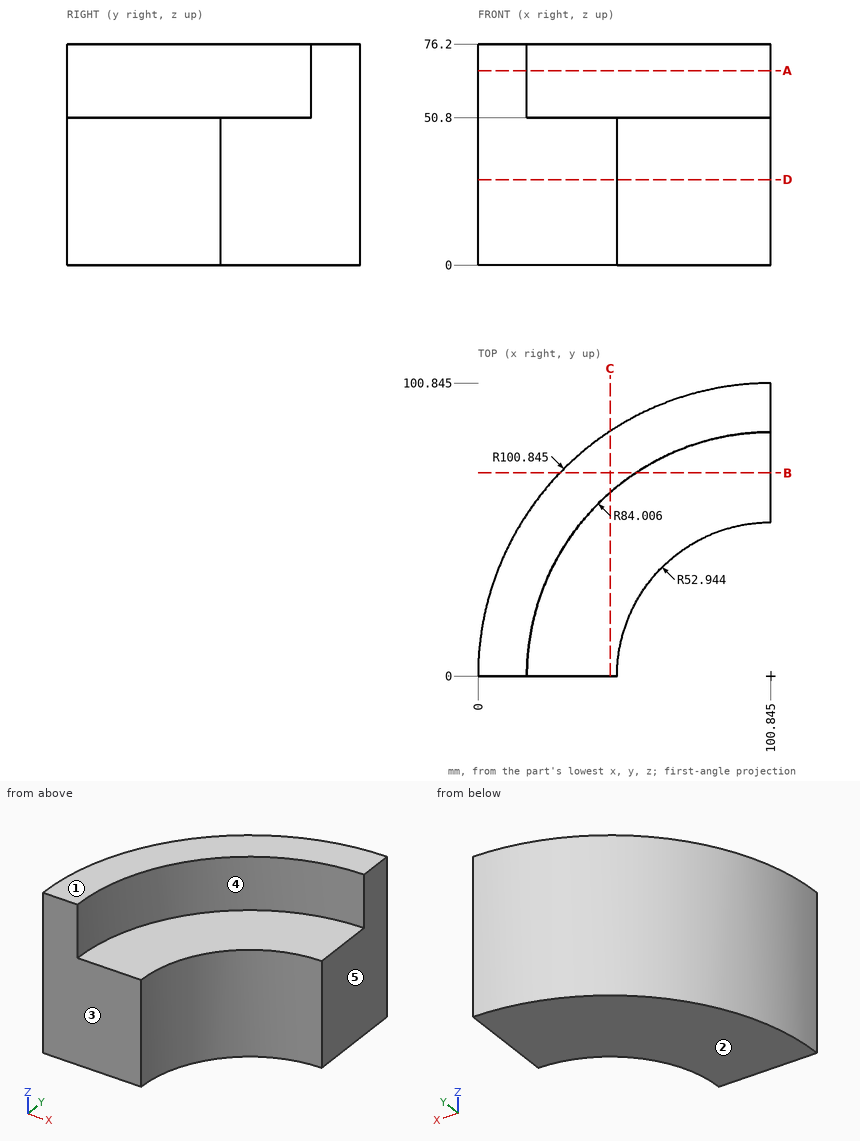
Can you work these out from the drawing? Everything is in mm from the part's minimum corner. A direction names the side the tool comes from. Round coordinates to 2 decimals unless told otherwise and drop trailing zeros. Write each loop counter-clockwise with the first axis right and the second up, starting at its lowest first coordinate (ties: lowest second). Pieces come first, ordered by that corner, then holes.
1. If we mould it in two halves opening along Z, with no side actions, what happens to the marked faces 1, 2 and 3? For each: released by +Z, released by -Z, zero draft, split by the parting line, or undercut.
2. For the marked faces 4 and 5, which set-ups out of +Z, -Z, +X, -X, +Y, -Y let a thin tool reach every point of the face, with its end or its side?
3. Suppose I cut it at C-C (x = 45.5). List the corners of the cut face in (y, z) for me.
4. Will these pins go through, and if not, where does the flat tip stop? pin 1 Ø1 at (x, y) = (50.5, 34) entering from +Z; pin 2 Ø4 at (y, z) = (67, 67) entering from +X; pin 3 Ø4 at (y, z) = (80.5, 39.5) entering from -X; pin 4 Ø25 at (x, y) = (38, 35) entering from +Z.
5. I need wall thicknesses on L1, parallel to Z at x = 59, y = 58; L2, parallel to Y at x = 68, z = 69 (1 decimal); L3, parallel to Y at x = 25.5, z = 27. Which ranges of each line are inside material? Lowest first, please.
6. Suppose I cut it at A-A (z = 67). List the corners of the cut face in (x, y) for me (1 decimal).
7. Suppose I cut it at D-D (z = 29.5). List the corners of the cut face in (x, y) for me (1 decimal).
8. Suppose I cut it at B-B (y = 70). List the corners of the cut face in (x, z) for me (1 decimal), and give its area (3 significant figures).
Answer sheet:
1. face 1: released by +Z
1. face 2: released by -Z
1. face 3: zero draft
2. face 4: +Z, +X, -Y
2. face 5: +Z, -Z, +X, +Y, -Y
3. outline: (0, 0) - (84.3, 0) - (84.3, 76.2) - (63.2, 76.2) - (63.2, 50.8) - (0, 50.8) - close
4. pin 1: stops at z = 50.8
4. pin 2: stops at x = 52.93
4. pin 3: stops at x = 37.54
4. pin 4: stops at z = 76.2
5. L1: z = 0 to 50.8
5. L2: y = 77.3 to 95.3
5. L3: y = 0 to 67.03
6. outline: (0, 0) - (16.8, 0) arc R84 cw to (100.8, 84) - (100.8, 100.8) arc R100.8 ccw to start
7. outline: (0, 0) - (47.9, 0) arc R52.9 cw to (100.8, 52.9) - (100.8, 100.8) arc R100.8 ccw to start
8. outline: (28.3, 0) - (100.8, 0) - (100.8, 50.8) - (54.4, 50.8) - (54.4, 76.2) - (28.3, 76.2) - close
8. area: 4,350 mm2
